Can you work these out from the model? Positions are in its coordinate system, mm. Coordinates: 2 decimals unless noted, no trailing zeros. Write each loop counter-clockwise with the first axis right and the second up, starting at its lowest first coordinate (ties: lowest second). Pieces come first, ordered by that corner, then holes. Notation, with made-up numbers: (42.25, 75) -> (82.25, 75) arc R14 cw to (82.25, 93) -> close; hole circle Ø4 at (-22.5, 50.5). An arc over 180 degrees is marked (long way). Use one line per item in the form item = value.
```python
from build123d import *

# Parameters (mm, degrees)
SKETCH_R       = 2
PAD_DEPTH      = 6
CYLINDER_R     = 3.7
CYLINDER_DEPTH = 10


with BuildPart() as part:
    # Sketch → Pad (new body)
    with BuildSketch(Plane.XY):
        with BuildLine():
            ThreePointArc((2.9e-05, 5), (-5, 1e-05), (1e-05, -5))
            Line((1e-05, -5), (20.00001, -5))
            ThreePointArc((20.00001, -5), (25.000039, -1e-05), (20.000029, 5))
            Line((2.9e-05, 5), (20.000029, 5))
        make_face()
        Circle(SKETCH_R, mode=Mode.SUBTRACT)
        with Locations((20.000039, 0)):
            Circle(SKETCH_R, mode=Mode.SUBTRACT)
    extrude(amount=PAD_DEPTH)

    # Cylinder → Cylinder (cut)
    with BuildSketch(Plane(origin=(10, 5, 0), x_dir=(1, 0, 0), z_dir=(0, -1, 0))):
        Circle(CYLINDER_R)
    extrude(amount=CYLINDER_DEPTH, mode=Mode.SUBTRACT)


solid = part.part
```
Q1. Suppose I cut it at C-C (x = 19.5). Write out the boundary of the cut face in (y, z), then the cut area to 3 significant figures.
Return value:
outline = (-5, 0) -> (-1.94, 0) -> (-1.94, 6) -> (-5, 6) -> close; (1.94, 0) -> (5, 0) -> (5, 6) -> (1.94, 6) -> close
area = 36.8 mm2
Q2. If I drill on line 1 (Y direction, x = 0, z = 1.2); line 2 (X direction, y = -1, z = 5.35); line 3 (X direction, y = -1.5, z = 4.8), over which ranges is the centre line in solid material (lowest first)? Write a range as from..to.
Return value:
line_1 = -5..-2, 2..5
line_2 = -4.9..-1.73, 1.73..18.27, 21.73..24.9
line_3 = -4.77..-1.32, 1.32..18.68, 21.32..24.77
Q3. Suppose I cut it at D-D (z = 3.4). Write out the boundary of the cut face in (x, y).
Return value:
outline = (0, -5) -> (8.54, -5) -> (8.54, 5) -> (0, 5) arc R5 ccw to start; (11.46, -5) -> (20, -5) arc R5 ccw to (20, 5) -> (11.46, 5) -> close; hole circle Ø4 at (0, 0); hole circle Ø4 at (20, 0)
Q4. Will this pin go through, and if not, where does the flat tip stop? pin 1 (4 mm diameter, centred on x = 9.5, y = 1, fed in from -Z).
Return value:
pin_1 = 2.73
Q5. Thinking about a two-plate mould opening in X: for faces 1 (the cylindrical face through (10.1, 0.1, 3.7)), 2 (the cylindrical face through (-5, 0, 3)), 3 (the flat face through (18, 1, 0)), 4 (the cylindrical face through (0, -2, 3)), which applies, released by +X, released by -X, zero draft, split by the parting line, or undercut?
Return value:
face_1 = undercut
face_2 = released by -X
face_3 = zero draft
face_4 = undercut
Q6. Suppose I cut it at B-B (z = 1.85). Write out the boundary of the cut face in (x, y), then the cut area to 3 significant figures.
Return value:
outline = (0, -5) -> (6.8, -5) -> (6.8, 5) -> (0, 5) arc R5 ccw to start; (13.2, -5) -> (20, -5) arc R5 ccw to (20, 5) -> (13.2, 5) -> close; hole circle Ø4 at (0, 0); hole circle Ø4 at (20, 0)
area = 189 mm2
Q7. Suppose I cut it at A-A (y = 0). Write out the boundary of the cut face in (x, z).
Return value:
outline = (-5, 0) -> (-2, 0) -> (-2, 6) -> (-5, 6) -> close; (2, 0) -> (6.3, 0) arc R3.7 cw to (13.7, 0) -> (18, 0) -> (18, 6) -> (2, 6) -> close; (22, 0) -> (25, 0) -> (25, 6) -> (22, 6) -> close
